```python
from build123d import *

# Parameters (mm, degrees)
SKETCH1_R                = 14
SKETCH1_R_2              = 10
BOSS_EXTRUDE1_DEPTH      = 20
BOSS_EXTRUDE2_REACH      = 61.262
BOSS_EXTRUDE2_END_RADIUS = 14
SKETCH4_W                = 10
SKETCH4_H                = 30
FILLET1_R                = 15
CUT_EXTRUDE1_REACH       = 50.59
SKETCH5_R                = 3


with BuildPart() as part:
    # Sketch1 → Boss-Extrude1 (new, symmetric)
    with BuildSketch(Plane.XY):
        Circle(SKETCH1_R)
        Circle(SKETCH1_R_2, mode=Mode.SUBTRACT)
    extrude(amount=BOSS_EXTRUDE1_DEPTH, both=True)

    # Boss-Extrude2: up to this cylinder (the profile starts outside it)
    boss_extrude2_end = Plane(origin=(0, 0, 0), z_dir=(0, 0, -1)) * Cylinder(BOSS_EXTRUDE2_END_RADIUS, 151.524, mode=Mode.PRIVATE)
    # Sketch4 → Boss-Extrude2 (add, up to the surface)
    with BuildSketch(Plane(origin=(0, 40, 0), x_dir=(1, 0, 0), z_dir=(0, 1, 0)), mode=Mode.PRIVATE) as boss_extrude2_sk1:
        Rectangle(SKETCH4_W, SKETCH4_H)
    boss_extrude2_tool1 = extrude(boss_extrude2_sk1.sketch, amount=-BOSS_EXTRUDE2_REACH, mode=Mode.PRIVATE) - boss_extrude2_end
    add(boss_extrude2_tool1.solids().sort_by_distance((0, 40, 0))[0])

    # Fillet1
    fillet1_edges = [part.edges().sort_by_distance(p)[0] for p in [
        (0, 40, 15),
        (0, 40, -15),
    ]]
    fillet(fillet1_edges, radius=FILLET1_R - 0.0001)  # a hair under: the kernel refuses the full size

    # Sketch5 → Cut-Extrude1 (cut, up to next)
    with BuildSketch(Plane.ZY.offset(5), mode=Mode.PRIVATE) as cut_extrude1_sk1:
        with Locations((0, 25)):
            Circle(SKETCH5_R)
    cut_extrude1_tool1 = extrude(cut_extrude1_sk1.sketch, amount=-CUT_EXTRUDE1_REACH, mode=Mode.PRIVATE) & part.part
    add(cut_extrude1_tool1.solids().sort_by_distance((-5, 25, 0))[0], mode=Mode.SUBTRACT)


solid = part.part
```
Source: CAD feature listing. Evaluate the final solid. Frame: model axes, mm. Give positions to 0.01 mm unless a question says otherwise; leave off trailing zeros. Loops run counter-clockwise (first coordinate to the right, second up) from the corner with the lowest first, then second, coordinate; pieces in that order, holes last. Notation, with made-up numbers: (21, 44) -> (48, 44) arc R21 cw to (48, 61) -> close; hole circle Ø6 at (-28, -31.5). An arc over 180 degrees is marked (long way). Put each result on its own line as item: value. Start each with the question number.
1) Cut plane C-C (z = -2). Return loops of the section in (x, y).
2) Contact query for flat-ended pins moving along their axis: P1, Ø12, axis at y = 5, z = 8, coming from the +X side; P2, Ø4, axis at x = -7.5, z = 0, coming from the -Y side; P3, Ø8, axis at y = 9.5, z = 14.5, coming from the +X side; P4, Ø3, axis at y = 25, z = 8, coming from the -X side. Output: stop coordinate, or through.
3) Cut plane B-B (y = 0). Return loops of the section in (x, z), then the cut area to 3 significant figures.
4) Cut plane D-D (x = 7). Return loops of the section in (y, z), then the cut area to 3 significant figures.
5) Draft query along X for faces 1 (the face through (-2.17, -9.76, -0.28)), 2 (the face through (-3, 10, 20)), 3 (the face through (-5, 27, -3)), 4 (the face through (5, 27, -3)). Return one class per face: released by +X, released by -X, zero draft, split by the parting line, or undercut.
6) Cut plane A-A (x = 0). State how many separate pieces and enclosed holes the cut face has, then the cut area to 3 significant figures.
7) Material intervals for probe 1 along Y at (x, z) = (-1.75, 2.5); probe 2 along Y at (x, z) = (0, 2); probe 3 along X at (y, z) = (-7.5, 10.5), sorted ascending.
Results are:
1. outline: (-5, 13.08) arc R14 ccw (long way) to (5, 13.08) -> (5, 22.76) -> (-5, 22.76) -> close; (-5, 27.24) -> (5, 27.24) -> (5, 39.87) -> (-5, 39.87) -> close; hole circle Ø20 at (0, 0)
2. P1: stops at x = 14
2. P2: stops at y = -12.87
2. P3: stops at x = 12.87
2. P4: stops at x = -5
3. outline: (-14, -20) -> (-10, -20) -> (-10, 20) -> (-14, 20) -> close; (10, -20) -> (14, -20) -> (14, 20) -> (10, 20) -> close
3. area: 320 mm2
4. outline: (-12.12, -20) -> (-7.14, -20) -> (-7.14, 20) -> (-12.12, 20) -> close; (7.14, -20) -> (12.12, -20) -> (12.12, 20) -> (7.14, 20) -> close
4. area: 399 mm2
5. face 1: undercut
5. face 2: zero draft
5. face 3: released by -X
5. face 4: released by +X
6. separate pieces: 2
6. enclosed holes: 1
6. area: 975 mm2
7. probe 1: y = -13.89 to -9.85, 9.85 to 23.34, 26.66 to 39.79
7. probe 2: y = -14 to -10, 10 to 22.76, 27.24 to 39.87
7. probe 3: x = -11.82 to -6.61, 6.61 to 11.82
